The listing builds one solid part. Answer for the finished solid, in the listing's coordinates (mm). A direction names the side the tool comes from. Give positions to 0.01 mm unless a question says otherwise; leave off trailing zeros. Loops run counter-clockwise (first coordinate to the right, second up) from the corner with the lowest first, then second, coordinate; pieces in that order, holes last. Notation, with made-up numbers: M -37,-15.5 L -19,-15.5 A5 ccw -19,-9.5 Z; hole C 30,30.25 d4. An arc over 180 degrees is marked long. Use one line per item in the form item = value. Start each with the question number.
1. Each of these flat-tipped pins is pushed along its axis until it touches: pin 1 Ø0.6 at (x, z) = (0, -15) entering from -Y; pin 2 Ø2 at (x, z) = (12.5, -11) entering from +Y; pin 3 Ø0.7 at (x, y) = (5.5, 12) entering from +Z; pin 4 Ø1.2 at (x, y) = (6, 12.5) entering from -Z. Where does it stop, or does it pass through?
2. For faces 1 (the face through (6, 12, 2.05)), 2 (the face through (0, 13, 2.1)), 3 (the face through (14, 0, -5)), determine the directions among +Z, -Z, +X, -X, +Y, -Y from which every point of the face is accessible in a straight line to the end or side of a thin tool.
3. The part is cut by section B-B (y = 7.5). Write down the section's boundary in (x, z), and give its area (3 significant figures).
4. The part is cut by section D-D (z = -15). Write down the section's boundary in (x, y), and give its area (3 significant figures).
5. The part is cut by section A-A (x = 0). Write down the section's boundary in (y, z).
6. The mould has two halves that part along Z. Classify faces 4 (the face through (0, 16, 3)), 5 (the face through (-16.108, 7.888, -3.577)), 6 (the face through (-6.35, 14.32, 0.05)): released by +Z, released by -Z, zero draft, split by the parting line, or undercut.
7. Straight lines are drawn through the part: line 1 (X direction, y = 0.8, z = 0); line 2 (X direction, y = 14.9, z = 0); line 3 (X direction, y = 12.5, z = 0). For each, find the intervals that lie inside material, in ascending order. Write a range as from..to.
8. The part is cut by section C-C (y = 2.5). Write down the section's boundary in (x, z), and give its area (3 significant figures).
from build123d import *

# Parameters (mm, degrees)
SKETCH_1_R               = 16.5
EXTRUDE_1_DEPTH          = 16
SKETCH_2_R               = 14.25
CUT_EXTRUDE_1_DEPTH      = 5.1
SKETCH_3_R               = 9.5
CUT_EXTRUDE_2_DEPTH      = 5
CUT_EXTRUDE_3_DEPTH      = 29.293108702
CUT_EXTRUDE_START        = -14
CUT_EXTRUDE_4_DEPTH      = 3.9
SKETCH_6_R               = 0.4
CUT_EXTRUDE_5_DEPTH      = 2
SKETCH_7_R               = 0.4
CUT_EXTRUDE_6_DEPTH      = 3
PATTERN_CIRCULAR_1_COUNT = 4
CUT_EXTRUDE_START_2      = -10.1
CUT_EXTRUDE_7_DEPTH      = 10.1


# Read off the part's stored shape, not the designer's step: 切除-拉伸4
with BuildPart() as part:
    # 草图1 → 凸台-拉伸1 (new body)
    with BuildSketch(Plane(origin=(0, 0, 0), x_dir=(1, 0, 0), z_dir=(0, 1, 0))):
        with Locations(Location((0, 0, 0), (0, 0, 270))):
            Circle(SKETCH_1_R)
    extrude(amount=EXTRUDE_1_DEPTH)

    # 草图2 → 切除-拉伸1 (cut)
    with BuildSketch(Plane(origin=(0, 0, 0), x_dir=(-1, 0, 0), z_dir=(0, -1, 0))):
        with Locations(Location((0, 0, 0), (0, 0, 90))):
            Circle(SKETCH_2_R)
    extrude(amount=-CUT_EXTRUDE_1_DEPTH, mode=Mode.SUBTRACT)

    # 草图3 → 切除-拉伸2 (cut)
    with BuildSketch(Plane.XZ.offset(-5.1)):
        with Locations(Location((0, 0, 0), (0, 0, 270))):
            Circle(SKETCH_3_R)
    extrude(amount=-CUT_EXTRUDE_2_DEPTH, mode=Mode.SUBTRACT)

    # 草图4 → 切除-拉伸3 (cut, through all)
    with BuildSketch(Plane.XZ):
        with BuildLine():
            ThreePointArc((-2.15, 0), (-2.76507576, 1.48492424), (-4.25, 2.1))
            Line((-4.25, 2.1), (-4.25, -2.1))
            ThreePointArc((-4.25, -2.1), (-2.76507576, -1.48492424), (-2.15, 0))
        make_face()
        with BuildLine():
            Line((-4.25, -2.1), (-4.25, 2.1))
            ThreePointArc((-4.25, 2.1), (-6.35, 0), (-4.25, -2.1))
        make_face()
        with BuildLine():
            ThreePointArc((4.25, -2.1), (2.15, 0), (4.25, 2.1))
            Line((4.25, 2.1), (-4.25, 2.1))
            ThreePointArc((-4.25, 2.1), (-2.76507576, 1.48492424), (-2.15, 0))
            ThreePointArc((-2.15, 0), (-2.76507576, -1.48492424), (-4.25, -2.1))
            Line((-4.25, -2.1), (4.25, -2.1))
        make_face()
        with BuildLine():
            ThreePointArc((6.35, 0), (5.73492424, 1.48492424), (4.25, 2.1))
            Line((4.25, 2.1), (4.25, -2.1))
            ThreePointArc((4.25, -2.1), (5.73492424, -1.48492424), (6.35, 0))
        make_face()
        with BuildLine():
            Line((4.25, -2.1), (4.25, 2.1))
            ThreePointArc((4.25, 2.1), (2.15, 0), (4.25, -2.1))
        make_face()
    extrude(amount=-CUT_EXTRUDE_3_DEPTH, mode=Mode.SUBTRACT)

    # 切除-拉伸4 outline → 切除-拉伸4 (cut)
    with BuildSketch(Plane.XZ.offset(CUT_EXTRUDE_START)):
        with BuildLine():
            ThreePointArc((7.15, -2.05), (9.2, 0), (7.15, 2.05))
            Line((7.15, 2.05), (4.705521679, 2.05))
            ThreePointArc((4.705521679, 2.05), (6.35, 0), (4.705521679, -2.05))
            Line((4.705521679, -2.05), (7.15, -2.05))
        make_face()
        with BuildLine():
            ThreePointArc((-4.705521679, -2.05), (-6.35, 0), (-4.705521679, 2.05))
            Line((-4.705521679, 2.05), (-7.15, 2.05))
            ThreePointArc((-7.15, 2.05), (-9.2, 0), (-7.15, -2.05))
            Line((-7.15, -2.05), (-4.705521679, -2.05))
        make_face()
    extrude(amount=CUT_EXTRUDE_4_DEPTH, mode=Mode.SUBTRACT)

    # 草图6 → 切除-拉伸5 (cut)
    with BuildSketch(Plane.XZ.offset(-14)):
        with Locations(Location((7.7, 0, 0), (0, 0, 270))):
            Circle(SKETCH_6_R)
        with Locations(Location((-7.7, 0, 0), (0, 0, 270))):
            Circle(SKETCH_6_R)
    extrude(amount=-CUT_EXTRUDE_5_DEPTH, mode=Mode.SUBTRACT)

    # 草图7 → 切除-拉伸6 (cut)
    with BuildSketch(Plane.XZ):
        with Locations(Location((15, 0, 0), (0, 0, 270))):
            Circle(SKETCH_7_R)
    cut_extrude_6 = extrude(amount=-CUT_EXTRUDE_6_DEPTH, mode=Mode.SUBTRACT)

    # 阵列(圆周)1: 切除-拉伸6 ×4 about axis
    pattern_circular_1_axis = Axis((0, 0, 0), (0, 1, 0))
    for i in range(1, PATTERN_CIRCULAR_1_COUNT):
        add(cut_extrude_6.rotate(pattern_circular_1_axis, i * 360 / PATTERN_CIRCULAR_1_COUNT), mode=Mode.SUBTRACT)

    # 草图8 → 切除-拉伸7 (cut)
    with BuildSketch(Plane.XZ.offset(CUT_EXTRUDE_START_2)):
        with BuildLine():
            Line((-14.03351048, 2.474486532), (0, 0))
            Line((0, 0), (-2.474486532, 14.03351048))
            ThreePointArc((-2.474486532, 14.03351048), (-10.076271632, 10.076271632), (-14.03351048, 2.474486532))
        make_face()
        with BuildLine():
            Line((-15.018318233, 2.648134709), (-14.03351048, 2.474486532))
            ThreePointArc((-14.03351048, 2.474486532), (-10.076271632, 10.076271632), (-2.474486532, 14.03351048))
            Line((-2.474486532, 14.03351048), (-2.648134709, 15.018318233))
            ThreePointArc((-2.648134709, 15.018318233), (-10.783378413, 10.783378413), (-15.018318233, 2.648134709))
        make_face()
    extrude(amount=CUT_EXTRUDE_7_DEPTH, mode=Mode.SUBTRACT)


solid = part.part
Derived:
q1.pin_1 = 3
q1.pin_2 = 16
q1.pin_3 = 15.68
q1.pin_4 = -15.59
q2.face_1 = -Y
q2.face_2 = +Y, -Y
q2.face_3 = +Z, -Z, +X, -X, -Y
q3.outline = C 0,0 d33; hole M -15.02,2.65 L -9.36,1.65 A9.5 ccw long -1.65,9.36 L -2.65,15.02 A15.25 ccw Z
q3.area = 485 mm2
q4.outline = M -6.87,0 L -0.4,0 L -0.4,3 L 0.4,3 L 0.4,0 L 6.87,0 L 6.87,16 L -6.87,16 Z
q4.area = 218 mm2
q5.outline = M 0,-16.5 L 16,-16.5 L 16,-2.1 L 10.1,-2.1 L 10.1,-9.5 L 5.1,-9.5 L 5.1,-14.25 L 0,-14.25 L 0,-14.6 L 3,-14.6 L 3,-15.4 L 0,-15.4 Z; M 0,14.25 L 5.1,14.25 L 5.1,9.5 L 10.1,9.5 L 10.1,2.1 L 16,2.1 L 16,16.5 L 0,16.5 L 0,15.4 L 3,15.4 L 3,14.6 L 0,14.6 Z
q6.face_4 = zero draft
q6.face_5 = split by the parting line
q6.face_6 = undercut
q7.line_1 = -16.5..-15.4, -14.6..-14.25, 14.25..14.6, 15.4..16.5
q7.line_2 = -16.5..-8.1, -7.3..-6.35, 6.35..7.3, 8.1..16.5
q7.line_3 = -16.5..-9.2, 9.2..16.5
q8.outline = C 0,0 d33; hole C -15,0 d0.8; hole M -15.02,2.65 L -14.03,2.47 A14.25 ccw long -2.47,14.03 L -2.65,15.02 A15.25 ccw Z; hole C 0,-15 d0.8; hole C 0,15 d0.8; hole C 15,0 d0.8
q8.area = 197 mm2
